```python
from build123d import *

# Parameters (mm, degrees)
F0_W     = 38.1607972085
F0_H     = 33.9049473405
F0_W_2   = 39.5794175565
F0_H_2   = 34.1886691749
F0_W_3   = 35.4654230177
F1_DEPTH = 25.4


with BuildPart() as f1:
    # F0 (on Front) → F1 (new body)
    with BuildSketch(Plane.XZ):
        with Locations((-19.0803986043, 16.9524736702)):
            Rectangle(F0_W, F0_H)
        Polygon((0, 68.2354792953), (0, 33.9049473405), (39.5794175565, 33.9049473405), (39.8631393909, 33.9049473405), (39.8631393909, 68.2354792953), align=None)
        with Locations((19.7897087783, 16.9524736702)):
            Rectangle(F0_W_2, F0_H)
        with Locations((-19.0803986043, -17.0943345875)):
            Rectangle(F0_W, F0_H_2)
        with Locations((19.7897087783, -17.0943345875)):
            Rectangle(F0_W_2, F0_H_2)
        with Locations((57.3121290654, -17.0943345875)):
            Rectangle(F0_W_3, F0_H_2)
    extrude(amount=F1_DEPTH)


solid = f1.part
```
Could you check a few things on this model? Use its own coordinates, in mm. A direction names the side the tool comes from. Round coordinates to 2 decimals unless told otherwise and drop trailing zeros. Loops run counter-clockwise (first coordinate to the right, second up) from the corner with the lowest first, then second, coordinate; pieces in that order, holes last. Notation, with made-up numbers: M 32.5,1.25 L 73.5,1.25 A14 cw 73.5,26.25 Z; hole C 27,-30 d6. An arc over 180 degrees is marked long. Write item = value, one per line.
1. Which directions (+Z, -Z, +X, -X, +Y, -Y) give clear straight access to the entire face, cutting with the end or side of a thin tool? Please do faces 5 (the face through (39.863, -13, 51)), 6 (the face through (18, -25.4, 6)), 7 (the face through (0, -13, 51)).
Results below:
face_5 = +Z, +X, +Y, -Y
face_6 = +Z, -Z, +X, -X, -Y
face_7 = +Z, -X, +Y, -Y
2. I want a section at B-B, the plane x = 49. Write out the boundary of the cut face in (y, z).
Results below:
outline = M -25.4,-34.19 L 0,-34.19 L 0,0 L -25.4,0 Z
3. Will these pins go through, and if not, where does the flat tip stop? P1, Ø4, axis at x = -9.5, z = -6, coming from the +Y side; P2, Ø2, axis at x = 62.5, y = -8.5, coming from the +Z side; P3, Ø7.5, axis at y = -9.5, z = 16, coming from the +X side; P4, Ø3, axis at y = -13, z = 52.5, coming from the -X side.
Results below:
P1 = 0
P2 = 0
P3 = 39.58
P4 = 0
4. I want a section at A-A, the plane y = -23.5. Write out the boundary of the cut face in (x, z), and give its area (3 significant figures).
Results below:
outline = M -38.16,-34.19 L 75.04,-34.19 L 75.04,0 L 39.58,0 L 39.58,33.9 L 39.86,33.9 L 39.86,68.24 L 0,68.24 L 0,33.9 L -38.16,33.9 Z
area = 7,870 mm²
5. Thinking about a two-plate mould opening in Z: for faces 1 (the face through (-19, -13, 33.905)), 2 (the face through (18, -13, -34.189)), 3 (the face through (39.579, -13, 17)), 4 (the face through (-38.161, -13, 0)), which applies, +Z half, -Z half, draft (parallel to the pull), parting line (faces both ways), or undercut?
Results below:
face_1 = +Z half
face_2 = -Z half
face_3 = undercut
face_4 = draft
6. I need wall thicknesses on probe 1 along X at (y, z) = (-16.25, 54); probe 2 along Z at (x, y) = (-33, -17.5); probe 3 along X at (y, z) = (-15.75, 15). Which ranges of each line are inside material? Lowest first, please.
Results below:
probe_1 = 0 to 39.86
probe_2 = -34.19 to 33.9
probe_3 = -38.16 to 39.58
7. I want a section at C-C, the plane z = 12. Write out the boundary of the cut face in (x, y), and give its area (3 significant figures).
Results below:
outline = M -38.16,-25.4 L 39.58,-25.4 L 39.58,0 L -38.16,0 Z
area = 1,970 mm²
